Here's how the part is built. I have some questions about the finished solid (model axes, mm). Face numbers are marked on the shaded views. A direction names the side the tool comes from. Give positions to 0.01 mm unless a question says otherwise; leave off trailing zeros. Write each loop counter-clockwise with the first axis right and the second up, starting at its lowest first coordinate (ties: lowest second). Pieces come first, ordered by that corner, then holes. Notation, with made-up numbers: (-2, -14) - (15, -14) arc R32 ccw to (15, 21) - close; hole circle Ø11 at (1, 12). An arc over 180 degrees is marked (long way). Write each question's results on one line, items separated by ' | '. Start each with the question number.
Item 1: Will these pins go through, and if not, where does the flat tip stop? P1, Ø1.5, axis at y = -4.5, z = 6, coming from the +X side; P2, Ø4, axis at y = -2, z = 13, coming from the +X side; P3, Ø3, axis at x = -19, y = -3.5, coming from the +Z side; P4, Ø3, axis at x = -14.5, z = 10.5, coming from the -Y side.
Item 2: Please list where these lines run through material, in increasing order: line 1 along Y through (x, z) = (-11.5, 7.5); line 2 along Y through (x, z) = (-17.5, 6.5); line 3 along X through (y, z) = (1.5, 1).
Item 3: Suppose I cut it at D-D on y = 2.75. List the corners of the cut face in (x, z) for me.
Item 4: Suppose I cut it at A-A on x = -19. List the corners of the cut face in (y, z) for me, then the cut area to 3 significant figures.
Item 5: Suppose I cut it at B-B on y = -7. List the corners of the cut face in (x, z) for me, then the cut area to 3 significant figures.
Item 6: We'd pull the mould along Y, two halves only. Please class the marked faces 6, 7 and 8: +Y half, -Y half, draft (parallel to the pull), parting line (faces both ways), or undercut.
Item 7: Which directions (+Z, -Z, +X, -X, +Y, -Y) give clear straight access to the entire face, cutting with the end or side of a thin tool? Please do the marked faces 1, 2, 3, 4 and 5.
Item 8: Suppose I cut it at C-C on y = -2.75. List the corners of the cut face in (x, z) for me, then the cut area to 3 significant figures.
```python
from build123d import *
from OCP.BRepAlgoAPI import BRepAlgoAPI_Cut
from OCP.TopTools import TopTools_ListOfShape

# Parameters (mm, degrees)
CROQUIS1_W              = 23.5
CROQUIS1_H              = 5
CROQUIS1_W_2            = 20.5
CROQUIS1_H_2            = 2
SALIENTE_EXTRUIR1_DEPTH = 15
SALIENTE_EXTRUIR2_DEPTH = 7
CROQUIS3_W              = 10
CROQUIS3_H              = 6
CORTAR_EXTRUIR1_DEPTH   = 9.213203
REDONDEO1_START         = -5.854446225
REDONDEO1_DEPTH         = 9.213203436
REDONDEO1_2_DEPTH       = 9.213203436
REDONDEO1_3_DEPTH       = 0.946564521
REDONDEO1_START_2       = 2.41219269
REDONDEO1_4_DEPTH       = 0.946564521
REDONDEO1_5_DEPTH       = 9.213203436
REDONDEO1_START_3       = -2
REDONDEO1_6_OUTLINE_W   = 11
REDONDEO1_6_OUTLINE_H   = 2.5
REDONDEO1_6_DEPTH       = 2
REDONDEO1_START_4       = 15
REDONDEO1_7_OUTLINE_W   = 11
REDONDEO1_7_OUTLINE_H   = 2.5
REDONDEO1_7_DEPTH       = 2
REDONDEO2_R             = 1.5


with BuildPart() as part:
    # Croquis1 → Saliente-Extruir1 (new body)
    with BuildSketch(Plane.XY):
        with Locations((-10.25, 1)):
            Rectangle(CROQUIS1_W, CROQUIS1_H)
        with Locations((-10.25, 1)):
            Rectangle(CROQUIS1_W_2, CROQUIS1_H_2, mode=Mode.SUBTRACT)
    extrude(amount=SALIENTE_EXTRUIR1_DEPTH)

    # Croquis2 → Saliente-Extruir2 (add)
    with BuildSketch(Plane.XZ.offset(1.5)):
        Polygon((-10.25, 15), (-1.764718626, 6.514718626), (-8.279437252, 0), (-16.764718626, 8.485281374), align=None)
    extrude(amount=SALIENTE_EXTRUIR2_DEPTH)


with BuildPart() as cortar_extruir1_tool:
    # Croquis3 → Cortar-Extruir1 (new body)
    with BuildSketch(Plane(origin=(-4.139718626, 0, -4.139718626), x_dir=(-0.7071067811865468, 0, 0.7071067811865482), z_dir=(-0.7071067811865482, 0, -0.7071067811865468))):
        with Locations((11.854446225, -4.5)):
            Rectangle(CROQUIS3_W, CROQUIS3_H)
    extrude(amount=-CORTAR_EXTRUIR1_DEPTH)


with BuildPart() as part_1:
    add(part.part)

    # Cortar-Extruir1: cut by cortar_extruir1_tool, with a tolerance
    cortar_extruir1_stock = TopTools_ListOfShape()
    cortar_extruir1_stock.Append(part_1.part.wrapped)
    cortar_extruir1_tools = TopTools_ListOfShape()
    cortar_extruir1_tools.Append(cortar_extruir1_tool.part.wrapped)
    cortar_extruir1_cut = BRepAlgoAPI_Cut()
    cortar_extruir1_cut.SetArguments(cortar_extruir1_stock)
    cortar_extruir1_cut.SetTools(cortar_extruir1_tools)
    cortar_extruir1_cut.SetFuzzyValue(0.00001)
    cortar_extruir1_cut.Build()
    add(Compound.cast(cortar_extruir1_cut.Shape()).solids(), mode=Mode.REPLACE)

    # Redondeo1: read off the stored shape, not the designer's step
    # Redondeo1 outline → Redondeo1 (cut)
    with BuildSketch(Plane(origin=(0, 0, 0), x_dir=(0.707106781186546, 0, -0.707106781186549), z_dir=(0.707106781186549, 0, 0.707106781186546)).offset(REDONDEO1_START)):
        with BuildLine():
            Line((-17.854446225, -8.5), (-15.854446225, -8.5))
            ThreePointArc((-15.854446225, -8.5), (-17.268659787, -7.914213562), (-17.854446225, -6.5))
            Line((-17.854446225, -6.5), (-17.854446225, -8.5))
        make_face()
        with BuildLine():
            ThreePointArc((-5.854446225, -6.5), (-6.440232663, -7.914213562), (-7.854446225, -8.5))
            Line((-7.854446225, -8.5), (-5.854446225, -8.5))
            Line((-5.854446225, -8.5), (-5.854446225, -6.5))
        make_face()
    extrude(amount=REDONDEO1_DEPTH, mode=Mode.SUBTRACT)

    # Redondeo1 2 outline → Redondeo1 2 (add)
    with BuildSketch(Plane(origin=(0, 0, 0), x_dir=(0.707106781186546, 0, -0.707106781186549), z_dir=(0.707106781186549, 0, 0.707106781186546)).offset(REDONDEO1_START)):
        with BuildLine():
            Line((-14.854446225, -1.5), (-16.854446225, -1.5))
            Line((-16.854446225, -1.5), (-16.854446225, -3.5))
            ThreePointArc((-16.854446225, -3.5), (-16.268659787, -2.085786438), (-14.854446225, -1.5))
        make_face()
        with BuildLine():
            Line((-6.854446225, -3.5), (-6.854446225, -1.5))
            Line((-6.854446225, -1.5), (-8.854446225, -1.5))
            ThreePointArc((-8.854446225, -1.5), (-7.440232663, -2.085786438), (-6.854446225, -3.5))
        make_face()
        with BuildLine():
            ThreePointArc((-14.854446225, -7.5), (-16.268659787, -6.914213562), (-16.854446225, -5.5))
            Line((-16.854446225, -5.5), (-16.854446225, -7.5))
            Line((-16.854446225, -7.5), (-14.854446225, -7.5))
        make_face()
        with BuildLine():
            Line((-6.854446225, -7.5), (-6.854446225, -5.5))
            ThreePointArc((-6.854446225, -5.5), (-7.440232663, -6.914213562), (-8.854446225, -7.5))
            Line((-8.854446225, -7.5), (-6.854446225, -7.5))
        make_face()
    extrude(amount=REDONDEO1_2_DEPTH)

    # Redondeo1 3 outline → Redondeo1 3 (add)
    with BuildSketch(Plane(origin=(0, 0, 0), x_dir=(0.707106781186546, 0, -0.707106781186549), z_dir=(0.707106781186549, 0, 0.707106781186546)).offset(REDONDEO1_START)):
        with BuildLine():
            ThreePointArc((-19.854446225, -1.5), (-18.440232663, -2.085786438), (-17.854446225, -3.5))
            Line((-17.854446225, -3.5), (-17.854446225, -1.5))
            Line((-17.854446225, -1.5), (-19.854446225, -1.5))
        make_face()
    extrude(amount=REDONDEO1_3_DEPTH)

    # Redondeo1 4 outline → Redondeo1 4 (add)
    with BuildSketch(Plane(origin=(0, 0, 0), x_dir=(0.707106781186546, 0, -0.707106781186549), z_dir=(0.707106781186549, 0, 0.707106781186546)).offset(REDONDEO1_START_2)):
        with BuildLine():
            Line((-5.854446225, -1.5), (-5.854446225, -3.5))
            ThreePointArc((-5.854446225, -3.5), (-5.268659787, -2.085786438), (-3.854446225, -1.5))
            Line((-3.854446225, -1.5), (-5.854446225, -1.5))
        make_face()
    extrude(amount=REDONDEO1_4_DEPTH)

    # Redondeo1 5 outline → Redondeo1 5 (add)
    with BuildSketch(Plane(origin=(0, 0, 0), x_dir=(0.7071067811865471, 0, -0.707106781186548), z_dir=(0.707106781186548, 0, 0.707106781186547)).offset(REDONDEO1_START)):
        with BuildLine():
            Line((-5.854446225, -1.5), (-5.854446225, -3.5))
            ThreePointArc((-5.854446225, -3.5), (-5.268659787, -2.085786438), (-3.854446225, -1.5))
            Line((-3.854446225, -1.5), (-5.854446225, -1.5))
        make_face()
        with BuildLine():
            Line((-17.854446225, -3.5), (-17.854446225, -1.5))
            Line((-17.854446225, -1.5), (-19.854446225, -1.5))
            ThreePointArc((-19.854446225, -1.5), (-18.440232663, -2.085786438), (-17.854446225, -3.5))
        make_face()
    extrude(amount=REDONDEO1_5_DEPTH)

    # Redondeo1 6 outline → Redondeo1 6 (cut)
    with BuildSketch(Plane.XY.offset(REDONDEO1_START_3)):
        with Locations((-9.5, -2.75)):
            Rectangle(REDONDEO1_6_OUTLINE_W, REDONDEO1_6_OUTLINE_H)
    extrude(amount=REDONDEO1_6_DEPTH, mode=Mode.SUBTRACT)

    # Redondeo1 7 outline → Redondeo1 7 (cut)
    with BuildSketch(Plane.XY.offset(REDONDEO1_START_4)):
        with Locations((-9.5, -2.75)):
            Rectangle(REDONDEO1_7_OUTLINE_W, REDONDEO1_7_OUTLINE_H)
    extrude(amount=REDONDEO1_7_DEPTH, mode=Mode.SUBTRACT)

    # Redondeo2
    redondeo2_edges = [part_1.edges().sort_by_distance(p)[0] for p in [
        (-22, -1.5, 7.5),
        (-22, 3.5, 7.5),
        (1.5, 3.5, 7.5),
        (1.5, -1.5, 7.5),
    ]]
    fillet(redondeo2_edges, radius=REDONDEO2_R)


solid = part_1.part
```
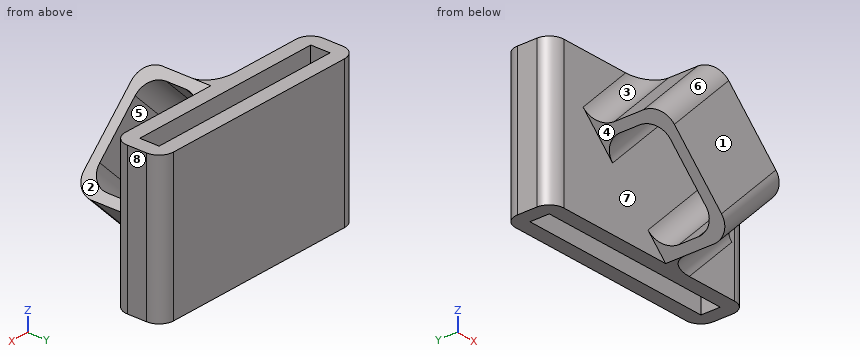
Checked values:
1) P1: stops at x = -1.76 | P2: stops at x = 1.5 | P3: passes through | P4: stops at y = -8.47
2) line 1: y = -8.5 to -7.5, -1.5 to 0, 2 to 3.5 | line 2: y = -1.5 to 0, 2 to 3.5 | line 3: x = -22 to -20.5, 0 to 1.5
3) outline: (-21.8, 0) - (1.3, 0) - (1.3, 15) - (-21.8, 15) - close
4) outline: (-1.5, 0) - (0, 0) - (0, 15) - (-1.5, 15) - close; (2, 0) - (3.5, 0) - (3.5, 15) - (2, 15) - close | area: 45.0 mm^2
5) outline: (-16.72, 8.44) - (-15.58, 7.3) - (-9.06, 13.81) - (-10.21, 14.96) - close; (-9.47, 1.19) - (-8.32, 0.04) - (-1.81, 6.56) - (-2.95, 7.7) - close | area: 29.7 mm^2
6) face 6: -Y half | face 7: undercut | face 8: draft
7) face 1: +Z, -Z, +X, -X, -Y | face 2: +Z, +X, -Y | face 3: +Z, -X, -Y | face 4: -Z, -X, -Y | face 5: none
8) outline: (-16.87, 8.59) - (-15.95, 7.67) - (-9.44, 14.19) - (-10.25, 15) - (-10.46, 15) - close; (-9.09, 0.81) - (-8.28, 0) - (-8.07, 0) - (-1.66, 6.41) - (-2.58, 7.33) - close | area: 23.8 mm^2
